Source: CAD feature listing. Evaluate the final solid. Frame: model axes, mm. A direction names the side the tool comes from. Round coordinates to 2 decimals unless told otherwise and drop trailing zeros. Loops run counter-clockwise (first coordinate to the right, second up) from the corner with the lowest first, then second, coordinate; pieces in that order, holes last. Notation, with made-up numbers: (20, 5.25) -> (76, 5.25) arc R18 cw to (76, 34.25) -> close; hole circle Ø10 at (8.25, 48). An arc over 180 degrees is marked (long way). Write item = value, one per line.
from build123d import *

# Parameters (mm, degrees)
F1_DEPTH     = 35
F3_D         = 4.5
F7_REACH     = 50.3610093633
F8_R         = 8
F10_DEPTH    = 4
F11_T4_DEPTH = 27.8083046081
F11_S5_R     = 12.5
F11_T6_DEPTH = 16


# Not quite as in the source:
# - a fillet or chamfer that OpenCascade refuses, or shapes differently, is made with other operations: its cross-section is extruded or revolved along the edge and cut away or added
# - a pattern or mirror of a feature is missing from the dataset's text; its kind, count and spacing are read off the source's solid


with BuildPart() as f1:
    # F0 (on Top) → F1 (new body, symmetric)
    with BuildSketch(Plane.XY):
        with BuildLine():
            Line((-24.5, 2), (-24.5, 0))
            Line((-24.5, 0), (-12.5, 0))
            Line((-12.5, 0), (-12.5, 13.5))
            ThreePointArc((-12.5, 13.5), (-8.8388347648, 22.3388347648), (0, 26))
            Line((0, 26), (0, 28))
            ThreePointArc((0, 28), (-10.2530483272, 23.7530483272), (-14.5, 13.5))
            Line((-14.5, 13.5), (-14.5, 2))
            Line((-14.5, 2), (-24.5, 2))
        make_face()
    extrude(amount=F1_DEPTH, both=True)

    # F3 (through all)
    with Locations(Plane(origin=(0, 2, 0), x_dir=(-1, 0, 0), z_dir=(0, 1, 0))):
        with Locations((19.5, -25), (19.5, 25)):
            Hole(F3_D / 2)

    # F4: F1 across plane


with BuildPart() as f1_1:
    add(f1.part)
    add(f1.part.mirror(Plane.YZ))

    f7_end = f1_1.faces().sort_by_distance((0, 26, 0))[0]
    # F6 (on offset) → F7 (cut, up to a face of the model that its end follows)
    with BuildSketch(Plane.XZ.offset(-29)):
        Polygon((0, 23), (0, 25), (-7.5, 25), (-7.5, 5), (-4.8855356313, 5), (-4.8855356313, 23), align=None)
    f7_long = extrude(amount=F7_REACH, mode=Mode.PRIVATE)
    f7 = split(f7_long, bisect_by=f7_end, keep=Keep.BOTTOM, mode=Mode.PRIVATE)
    add(f7, mode=Mode.SUBTRACT)

    # F7_copies: F7 across plane
    add(f7.mirror(Plane(origin=(0, 0, 0), x_dir=(0, 0, 1), z_dir=(1, 0, 0))), mode=Mode.SUBTRACT)

    # F8
    f8_edges = [f1_1.edges().sort_by_distance(p)[0] for p in [
        (-24.5, 1, -35),
        (24.5, 1, -35),
        (-24.5, 1, 35),
        (24.5, 1, 35),
    ]]
    fillet(f8_edges, radius=F8_R)

    # F9 (on face) → F10 (join)
    with BuildSketch(Plane.XY.offset(23)):
        with BuildLine():
            ThreePointArc((4.8855356313, 25.0057177783), (0, 26), (-4.8855356313, 25.0057177783))
            Line((-4.8855356313, 25.0057177783), (-4.8855356313, 23.0057177783))
            Line((-4.8855356313, 23.0057177783), (4.8855356313, 23.0057177783))
            Line((4.8855356313, 23.0057177783), (4.8855356313, 25.0057177783))
        make_face()
    extrude(amount=-F10_DEPTH)

    # F11: chamfer of 3 x 3.5 on 1 edges, made by hand


with BuildPart() as f11_tool2:
    # F11_s3 → F11_t4 (new body)
    with BuildSketch(Plane.YZ.offset(-13.9041523041)):
        Polygon((23.0057177783, 22.5), (26.0057177783, 19), (23.0057177783, 19), align=None)
    extrude(amount=F11_T4_DEPTH)

    # F11_s5 → F11_t6 (intersect, symmetric)
    with BuildSketch(Plane.XY.offset(20.8)):
        with Locations((0, 13.5)):
            Circle(F11_S5_R)
    extrude(amount=F11_T6_DEPTH, both=True, mode=Mode.INTERSECT)


with BuildPart() as f1_2:
    add(f1_1.part)

    # F11_t1: cut F11_tool2
    add(f11_tool2.part, mode=Mode.SUBTRACT)


solid = f1_2.part
1. Set-up query: faces 1 (the face through (-19, 2, 0)), 2 (the face through (19, 2, 0)), 3 (the face through (-19, 0, 0)), 4 (the face through (-22.094, 0.986, -32.719)), 5 (the face through (0, 26, 23)). Return all of +Z, -Z, +X, -X, +Y, -Y with unobstructed straight access to the full face (end or side cutting, diameter ignored); none if empty.
Evaluation:
face_1 = +Z, -Z, -X, +Y
face_2 = +Z, -Z, +X, +Y
face_3 = +Z, -Z, +X, -X, -Y
face_4 = -Z, -X, +Y, -Y
face_5 = +Y, -Y
2. Section query D-D (x = -3.5). Return the cut outline in (y, z), then the cut area to 3 significant figures.
Evaluation:
outline = (23.01, 22.5) -> (25.5, 19.59) -> (25.5, -35) -> (27.57, -35) -> (27.57, 23) -> (23.01, 23) -> close; (25.5, 25) -> (27.57, 25) -> (27.57, 35) -> (25.5, 35) -> close
area = 146 mm²
3. Mould query, pull axis Z, two halves, no side actions, for faces 6 (the face through (18.462, 0.986, 23.004)), 7 (the face through (22.219, 0.986, -32.594)), 8 (the face through (-12.5, 7, 0)). Classes: released by +Z, released by -Z, zero draft, split by the parting line, or undercut.
Evaluation:
face_6 = undercut
face_7 = released by -Z
face_8 = zero draft
4. Section query B-B (y = 11.5). Return the cut outline in (x, z), then the cut area to 3 significant figures.
Evaluation:
outline = (-14.5, -35) -> (-12.5, -35) -> (-12.5, 35) -> (-14.5, 35) -> close; (12.5, -35) -> (14.5, -35) -> (14.5, 35) -> (12.5, 35) -> close
area = 280 mm²
5. Section query C-C (x = -20). Return the cut outline in (y, z).
Evaluation:
outline = (0, -34.19) -> (2, -34.19) -> (2, -27.19) -> (0, -27.19) -> close; (0, -22.81) -> (2, -22.81) -> (2, 22.81) -> (0, 22.81) -> close; (0, 27.19) -> (2, 27.19) -> (2, 34.19) -> (0, 34.19) -> close
6. Contact query for flat-ended pins moving along their axis: pin 1 Ø3.5 at (y, z) = (26, 10.5) entering from +X; pin 2 Ø3 at (y, z) = (7, 19) entering from +X; pin 3 Ø3 at (x, z) = (8, 23.5) entering from -Y; pin 4 Ø4 at (x, z) = (-19.5, -25) entering from +Y. Output: stop coordinate, or through.
Evaluation:
pin_1 = 9.73
pin_2 = 14.5
pin_3 = 21.62
pin_4 = through
7. Section query A-A (z = -25). Return the cut outline in (x, y), then the cut area to 3 significant figures.
Evaluation:
outline = (-24.5, 0) -> (-21.75, 0) -> (-21.75, 2) -> (-24.5, 2) -> close; (-17.25, 0) -> (-12.5, 0) -> (-12.5, 13.5) arc R12.5 cw to (12.5, 13.5) -> (12.5, 0) -> (17.25, 0) -> (17.25, 2) -> (14.5, 2) -> (14.5, 13.5) arc R14.5 ccw to (-14.5, 13.5) -> (-14.5, 2) -> (-17.25, 2) -> close; (21.75, 0) -> (24.5, 0) -> (24.5, 2) -> (21.75, 2) -> close
area = 161 mm²
8. Line query: probe 1 along Z at (x, y) = (-19.5, 1.2); probe 2 along X at (y, z) = (3, -18); probe 3 along Y at (x, z) = (-15.5, -11). Output: solid intervals per line, ascending. Write a range as from..to.
Evaluation:
probe_1 = -34.42..-27.25, -22.75..22.75, 27.25..34.42
probe_2 = -14.5..-12.5, 12.5..14.5
probe_3 = 0..2
